```python
from build123d import *

# Parameters (mm, degrees)
F0_W     = 40
F0_H     = 10
F1_DEPTH = 3
F2_R     = 2
F3_DEPTH = 20
F4_DEPTH = 10
F5_DEPTH = 15


with BuildPart() as f1:
    # F0 (on Top) → F1 (new body)
    with BuildSketch(Plane.XY):
        Rectangle(F0_W, F0_H)
    extrude(amount=F1_DEPTH)

    # F2 (on face) → F3 (join)
    with BuildSketch(Plane.XY.offset(3)):
        with Locations((-14, 0)):
            Circle(F2_R)
        with Locations((14, 0)):
            Circle(F2_R)
    extrude(amount=F3_DEPTH)

    # F2 (on face) → F4 (join)
    with BuildSketch(Plane.XY.offset(3)):
        with Locations((-6, 0)):
            Circle(F2_R)
    extrude(amount=F4_DEPTH)

    # F2 (on face) → F5 (join)
    with BuildSketch(Plane.XY.offset(3)):
        with Locations((6, 0)):
            Circle(F2_R)
    extrude(amount=F5_DEPTH)


solid = f1.part
```
Model file for the job. Use its own axes, mm. A direction names the side the tool comes from. Give positions to 0.01 mm unless a question says otherwise; leave off trailing zeros. Order: outer loops, then holes, each group sorted by start corner. A loop starts at its lowest first (then second) coordinate and runs counter-clockwise, first axis right, second up.
1) Saw through at A-A, the plane x = -6. Write the cut outline in (y, z).
2) Wall check: probe 1 along X at (y, z) = (-1.5, 7.75); probe 2 along Z at (x, y) = (10, 0.5); probe 3 along X at (y, z) = (-1.25, 14). Give the ranges that are in metal, low to high.
3) Mould opens along X. For faces 1 (the cylindrical face through (-7.6, -1.2, 7.9)), 2 (the flat face through (-20, 0, 1)), 3 (the flat face through (0, -5, 1)) say: +X half, -X half, draft (parallel to the pull), parting line (faces both ways), or undercut.
4) Saw through at B-B, the plane z = 17. Write the cut outline in (x, y), then the cut area to 3 significant figures.
5) Pin check, flat tips, straight feed: pin 1 (3 mm diameter, centred on y = -4, z = 10.5, fed in from -X); pin 2 (3 mm diameter, centred on x = 0, y = -2, fed in from +Z); pin 3 (4 mm diameter, centred on x = 15, y = -3, fed in from +Z); pin 4 (3 mm diameter, centred on x = -5, y = 1, fed in from +Z). Stop position of each tip, or through.
6) 3-axis set-ups, long thin cutter, end or side, ignore diameter. For faces 4 (the cylindrical face through (4.4, -1.2, 10.4)), 5 (the flat face through (-6, 0, 13)), 6 (the flat face through (0, 0, 0)): which of +Z, -Z, +X, -X, +Y, -Y reach the whole face in a straight line?
7) Saw through at C-C, the plane z = 7. Write the cut outline in (x, y), then the cut area to 3 significant figures.
8) Saw through at D-D, the plane y = 0. Write the cut outline in (x, z), then the cut area to 3 significant figures.
Computed:
1. outline: (-5, 0) - (5, 0) - (5, 3) - (2, 3) - (2, 13) - (-2, 13) - (-2, 3) - (-5, 3) - close
2. probe 1: x = -15.32 to -12.68, -7.32 to -4.68, 4.68 to 7.32, 12.68 to 15.32
2. probe 2: z = 0 to 3
2. probe 3: x = -15.56 to -12.44, 4.44 to 7.56, 12.44 to 15.56
3. face 1: undercut
3. face 2: -X half
3. face 3: draft
4. outline: circle Ø4 at (-14, 0); circle Ø4 at (6, 0); circle Ø4 at (14, 0)
4. area: 37.7 mm2
5. pin 1: passes through
5. pin 2: stops at z = 3
5. pin 3: stops at z = 23
5. pin 4: stops at z = 13
6. face 4: +Z
6. face 5: +Z, +Y, -Y
6. face 6: -Z, +X, -X, +Y, -Y
7. outline: circle Ø4 at (-14, 0); circle Ø4 at (-6, 0); circle Ø4 at (6, 0); circle Ø4 at (14, 0)
7. area: 50.3 mm2
8. outline: (-20, 0) - (20, 0) - (20, 3) - (16, 3) - (16, 23) - (12, 23) - (12, 3) - (8, 3) - (8, 18) - (4, 18) - (4, 3) - (-4, 3) - (-4, 13) - (-8, 13) - (-8, 3) - (-12, 3) - (-12, 23) - (-16, 23) - (-16, 3) - (-20, 3) - close
8. area: 380 mm2
